Can you work these out from the drawing? Everything is in mm from the part's minimum corner. Coordinates: 2 decimals unless noted, no trailing zeros. Write each loop counter-clockwise with the first axis right and the second up, starting at its lowest first coordinate (ties: lowest second). Pieces come first, ordered by that corner, then holes. Notation, with made-up numbers: (1.25, 84) -> (49.25, 84) arc R17 cw to (49.25, 106) -> close; hole circle Ø3 at (28, -28). An arc over 180 degrees is marked (long way). Use CSV: the item, a comma, the result in double quotes. Start each with the question number.
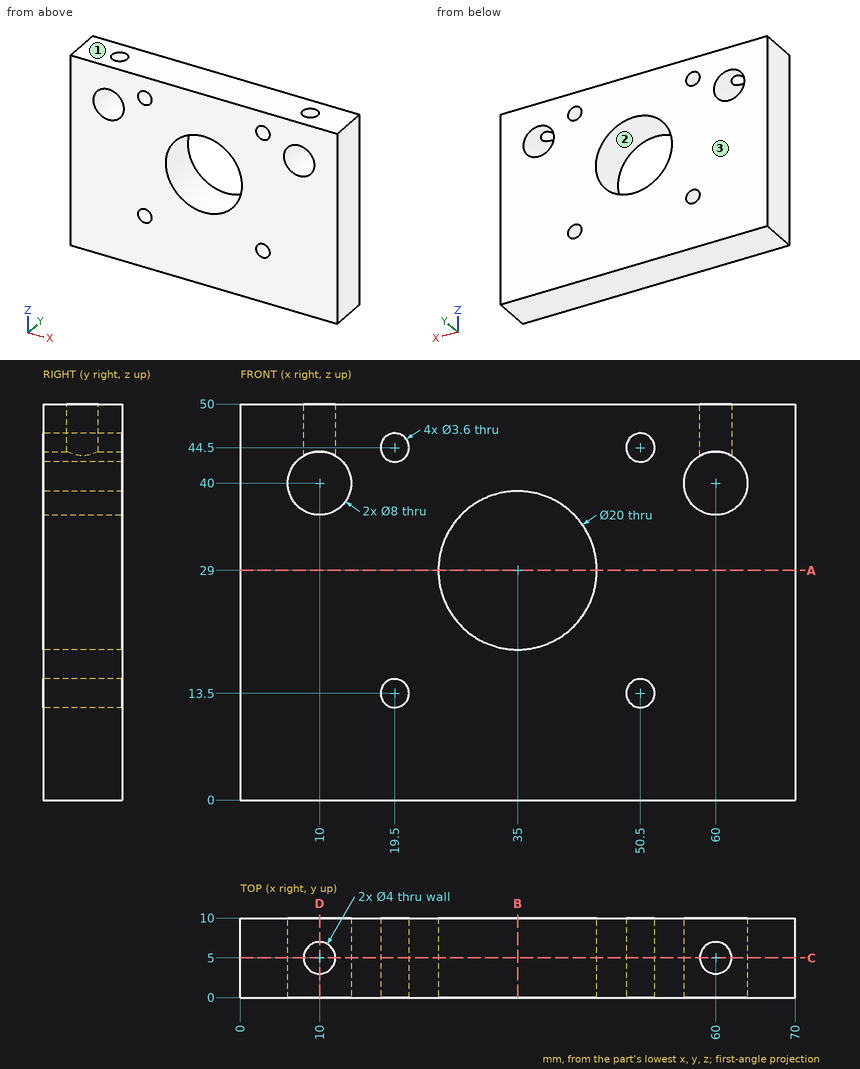
Item 1: I want a section at B-B on x = 35. Please give me the cut outline in (y, z).
Item 2: I want a section at D-D on x = 10. Please give me the cut outline in (y, z), then the cut area to 3 significant figures.
Item 3: I'm going to push flat-ended pins straight in: pin 1 (5 mm diameter, centred on y = 2, z = 9, fed in from -X); pin 2 (3 mm diameter, centred on x = 19.5, z = 13.5, fed in from -Y). Where does each tip first touch, or does it pass through?
Item 4: I want a section at C-C on y = 5. Please give me the cut outline in (x, z), then the cut area to 3 significant figures.
Item 5: Thinking about a two-plate mould opening in Z: for the marked faces 1, 2 and 3, which applies, +Z half, -Z half, draft (parallel to the pull), parting line (faces both ways), or undercut?
Item 6: If I drill on line 1 along Z through (x, y) = (19.5, 4); line 2 along X through (y, z) = (6.25, 40); line 3 along Z through (x, y) = (10, 8.25), over which ranges is the centre line in solid material (lowest first)?
Item 7: I want a section at A-A on z = 29. Please give me the cut outline in (x, y).
Geometry says:
1,outline,"(0, 0) -> (10, 0) -> (10, 19) -> (0, 19) -> close; (0, 39) -> (10, 39) -> (10, 50) -> (0, 50) -> close"
2,outline,"(0, 0) -> (10, 0) -> (10, 36) -> (0, 36) -> close; (0, 44) -> (3, 44) -> (3, 50) -> (0, 50) -> close; (7, 44) -> (10, 44) -> (10, 50) -> (7, 50) -> close"
2,area,"396 mm2"
3,pin 1,"x = 0"
3,pin 2,"through"
4,outline,"(0, 0) -> (70, 0) -> (70, 50) -> (62, 50) -> (62, 43.46) arc R4 cw (long way) to (58, 43.46) -> (58, 50) -> (12, 50) -> (12, 43.46) arc R4 cw (long way) to (8, 43.46) -> (8, 50) -> (0, 50) -> close; hole circle Ø3.6 at (19.5, 13.5); hole circle Ø3.6 at (19.5, 44.5); hole circle Ø20 at (35, 29); hole circle Ø3.6 at (50.5, 13.5); hole circle Ø3.6 at (50.5, 44.5)"
4,area,"3,000 mm2"
5,face 1,"+Z half"
5,face 2,"undercut"
5,face 3,"draft"
6,line 1,"0 to 11.7, 15.3 to 42.7, 46.3 to 50"
6,line 2,"0 to 6, 14 to 56, 64 to 70"
6,line 3,"0 to 36, 44 to 50"
7,outline,"(0, 0) -> (25, 0) -> (25, 10) -> (0, 10) -> close; (45, 0) -> (70, 0) -> (70, 10) -> (45, 10) -> close"
